Autodesk Inventor part; units mm, degrees
ref_plane "YZ Plane" through (0, 0, 0) normal (1, 0, 0) x (0, 1, 0)
ref_plane "XZ Plane" through (0, 0, 0) normal (0, 1, 0) x (-1, 0, 0)
ref_plane "XY Plane" through (0, 0, 0) normal (0, 0, 1) x (1, 0, 0)
sketch "Sketch1" plane through (0, 0, 0) normal (0, 0, 1) x (1, 0, 0)
  line L0 (-8, -0.5) -> (-13.542, -0.5)
  arc A0 (-8, -0.5) -> (-8, 0.5) centre (-8, 0) ccw
  line L1 (-8, 0.5) -> (-13.542, 0.5)
  arc A1 (-16.5, 3) -> (-13.542, 0.5) centre (-13.542, 3.5) ccw
  line L2 (-16.5, 3) -> (-16.5, 2)
  line L3 (-16.5, 2) -> (-18.5, 1.2721)
  line L4 (-18.5, 1.2721) -> (-18.5, 0.2721)
  line L5 (-18.5, 0.2721) -> (-16.5, 1)
  arc A2 (-13.542, -0.5) -> (-16.5, -3) centre (-13.542, -3.5) ccw
  line L6 (-22.2, 0) -> (3.7, 0) construction
  line L7 (0, -4.9) -> (0, 4.9) construction
  line L8 (-16.5, 1) -> (-16.5, -1)
  line L9 (-16.5, -1) -> (-18.5, -1.7279)
  line L10 (-18.5, -1.7279) -> (-18.5, -2.7279)
  line L11 (-18.5, -2.7279) -> (-16.5, -2)
  line L12 (-16.5, -2) -> (-16.5, -3)
  point P0 (0, 0)
  point P1 (-7.5, 0)
  dimension "d3" = 15
  dimension "d4" = 33
  dimension "d5" = 2
  dimension "d7" = 1
  dimension "d8" = 6
  dimension "d9" = 3
  dimension "d10" = 1
  dimension "d12" = 2
  dimension "d13" = 5.542
  dimension "d15" = 0.7279
  dimension "d16" = 70
revolve "Revolution1" add sketch "Sketch1" angle 360 about axis through (0, -10, 0) along (0, 1, 0)
properties part number "Sealingring"
CAD build for the part. Positions are in the model's coordinates, mm. Give positions to 0.01 mm unless a question says otherwise; leave off trailing zeros. Order: outer loops, then holes, each group sorted by start corner. A loop starts at its lowest first (then second) coordinate and runs counter-clockwise, first axis right, second up. Notation, with made-up numbers: (-20, 85.5) -> (-16, 85.5) arc R30 cw to (-16, 124.5) -> close; hole circle Ø9 at (77, 64.25). An arc over 180 degrees is marked (long way). Return JSON: item names as keys, results as strings.
Q1. Saw through at A-A (z = 0). Write the cut outline in (x, y), then the cut area to 3 significant figures.
Working result:
{"outline": "(-18.5, -2.73) -> (-16.5, -2) -> (-16.5, -3) arc R3 cw to (-13.54, -0.5) -> (-8, -0.5) arc R0.5 ccw to (-8, 0.5) -> (-13.54, 0.5) arc R3 cw to (-16.5, 3) -> (-16.5, 2) -> (-18.5, 1.27) -> (-18.5, 0.27) -> (-16.5, 1) -> (-16.5, -1) -> (-18.5, -1.73) -> close; (8, -0.5) -> (13.54, -0.5) arc R3 cw to (16.5, -3) -> (16.5, -2) -> (18.5, -2.73) -> (18.5, -1.73) -> (16.5, -1) -> (16.5, 1) -> (18.5, 0.27) -> (18.5, 1.27) -> (16.5, 2) -> (16.5, 3) arc R3 cw to (13.54, 0.5) -> (8, 0.5) arc R0.5 ccw to start", "area": "33.1 mm²"}
Q2. Mould opens along Y. For faces 1 (the face through (-15.24, -0.01, 6.32)), 2 (the face through (-6, 0.5, -6)), 3 (the face through (-6, -0.5, -6)) say: pulls with the +Y half, pulls with the -Y half, needs draft (parallel to the pull), parting line crosses it, or undercut.
Working result:
{"face 1": "undercut", "face 2": "pulls with the +Y half", "face 3": "pulls with the -Y half"}
Q3. Drill centre lines: line 1 (Y direction, x = -10, z = 9); line 2 (X direction, y = -1.75, z = 3.5); line 3 (Z direction, x = 7.5, y = 1.25). Where is each one in solid material? Low to high.
Working result:
{"line 1": "-0.5 to 0.5", "line 2": "-18.17 to -15.59, 15.59 to 18.17", "line 3": "-16.91 to -13.59, 13.59 to 16.91"}
Q4. Saw through at B-B (x = 0). Write the cut outline in (y, z), then the cut area to 3 significant figures.
Working result:
{"outline": "(-3, -16.5) -> (-2, -16.5) -> (-2.73, -18.5) -> (-1.73, -18.5) -> (-1, -16.5) -> (1, -16.5) -> (0.27, -18.5) -> (1.27, -18.5) -> (2, -16.5) -> (3, -16.5) arc R3 cw to (0.5, -13.54) -> (0.5, -8) arc R0.5 ccw to (-0.5, -8) -> (-0.5, -13.54) arc R3 cw to start; (-3, 16.5) arc R3 cw to (-0.5, 13.54) -> (-0.5, 8) arc R0.5 ccw to (0.5, 8) -> (0.5, 13.54) arc R3 cw to (3, 16.5) -> (2, 16.5) -> (1.27, 18.5) -> (0.27, 18.5) -> (1, 16.5) -> (-1, 16.5) -> (-1.73, 18.5) -> (-2.73, 18.5) -> (-2, 16.5) -> close", "area": "33.1 mm²"}
Q5. Flat gauge pins, fed straight in: pin 1 (2 mm diameter, centred on y = -2.5, z = -2.5, fed in from -X); pin 2 (8 mm diameter, centred on x = 10.5, z = -1, fed in from +Y); pin 3 (13.5 mm diameter, centred on x = -6.5, z = 6, fed in from -Y). Where does each tip first touch, or does it go through?
Working result:
{"pin 1": "x = -18.44", "pin 2": "y = 0.67", "pin 3": "y = -1.31"}
